Part model, mm, in its own coordinate system. Face numbers are marked on the shaded views. A direction names the side the tool comes from. Round coordinates to 2 decimals unless told otherwise and drop trailing zeros. Write each loop counter-clockwise with the first axis right and the second up, starting at its lowest first coordinate (ties: lowest second). Pieces come first, ordered by that corner, then holes. Notation, with made-up numbers: (-2, -37.75) -> (24, -37.75) arc R7 cw to (24, -25.75) -> close; hole circle Ø5 at (60.5, 13). An arc over 180 degrees is marked (long way). Use CSV: the item, a comma, the result in double quotes. Start each with the question number.
Autodesk Inventor part; units mm, degrees
ref_plane "YZ Plane" through (0, 0, 0) normal (1, 0, 0) x (0, 1, 0)
ref_plane "XZ Plane" through (0, 0, 0) normal (0, 1, 0) x (-1, 0, 0)
ref_plane "XY Plane" through (0, 0, 0) normal (0, 0, 1) x (1, 0, 0)
sketch "Skizze1" plane through (0, 0, 0) normal (0, 0, 1) x (1, 0, 0)
  arc A0 (-8.1406, -4.7) -> (-8.6412, -3.7) centre (0, 0) ccw
  line L0 (-18.5, -6.7) -> (-8.3427, -6.7)
  line L1 (-18.5, -6.7) -> (-18.5, -4.7)
  line L2 (-18.5, -4.7) -> (-8.1406, -4.7)
  line L3 (-18.5, -1.7) -> (-18.5, -3.7)
  line L4 (-18.5, -3.7) -> (-8.6412, -3.7)
  line L5 (-18.5, -1.7) -> (-14.519, -1.7)
  arc A1 (-8.3427, -6.7) -> (-10.5682, 1.6741) centre (0, 0) ccw
  arc A2 (-14.519, -1.7) -> (-10.5682, 1.6741) centre (-14.519, 2.3) ccw
  point P0 (-10.5641, -1.7)
  dimension "d0" = 18.8
  dimension "d2" = 2
  dimension "d4" = 1
  dimension "d5" = 18.5
  dimension "d6" = 4
  dimension "d7" = 1.3
  dimension "d19" = 10.1573
  dimension "d26" = 4
extrude "Extrusion1" add sketch "Skizze1" along normal mid plane 14
sketch "Skizze2" plane through (-18.5, -1.7, 7) normal (0, 1, 0) x (1, 0, 0)
  circle A0 centre (3, 11) radius 1.65
  line L0 (0, 14) -> (3.981, 14)
  line L1 (0, 14) -> (0, 0)
  line L2 (0, 14) -> (0, 0) construction
  line L3 (0, 7) -> (7.2294, 7) construction
  circle A1 centre (3, 3) radius 1.65
  circle A2 centre (3, 11) radius 3
  circle A3 centre (3, 3) radius 3
  point P0 (18.5, 7)
  point P1 (9.0709, 16)
  point P2 (0, 3)
  point P3 (0, 0.6676)
  point P4 (0.6676, 16)
  point P5 (0, 11)
  point P6 (0, 10.6676)
  point P7 (3, 14)
  dimension "d10" = 3
  dimension "d11" = 3
  dimension "d12" = 3.3
  dimension "d20" = 6
extrude "Extrusion2" cut sketch "Skizze2" against normal through all both and the other way through all contours A0 | A1
fillet "Rundung2" radius 4 1 edges at (-8.3427, -6.7, 0)
fillet "Rundung3" radius 0.8 2 edges at (-8.6412, -3.7, 0) (-8.1406, -4.7, 0)
extrude "Extrusion4" cut sketch "Skizze2" along normal blind 10 contours A3 | A2
properties part number "Halterung_Akku_210403"
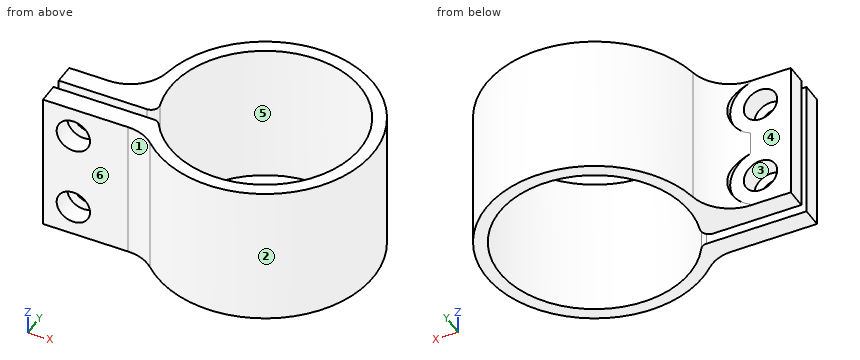
1. Band-saw the part on A-A (x = -15.5). List the corners of the cut face in (y, z).
2. Drill centre lines: line 1 along Z through (x, y) = (-15.5, -2.95); line 2 along X through (y, z) = (-3.1, -4); line 3 along X through (y, z) = (-5, 3). Where is each one in solid material? Low to high. Write a range as [from, to].
3. Band-saw the part on B-B (z = 4). List the corners of the cut face in (x, y), then the cut area to 3 significant figures.
4. Which spindle directions (+Z, -Z, +X, -X, +Y, -Y) get a long thin tool onto all of the face, cutting with end or side? Do the marked faces 4, 5 and 6. Say none if no direction does.
5. Pull direction X, two halves, no side cores. Call the marked faces 1, 2 and 3: released by +X, released by -X, zero draft, split by the parting line, or undercut.
6. Flat gauge pins, fed straight in: pin 1 (1.5 mm diameter, centred on y = 6.5, z = 5, fed in from -X); pin 2 (5 mm diameter, centred on x = 3, z = 4, fed in from +Y); pin 3 (5 mm diameter, centred on x = -5.5, z = -4.5, fed in from +Y). Where does each tip first touch, or does it go through?
7. Band-saw the part on D-D (x = -6.5). List the corners of the cut face in (y, z), then the cut area to 3 significant figures.
8. Band-saw the part on C-C (y = 2.25). List the corners of the cut face in (x, z), then the cut area to 3 significant figures.
Answers below:
1,outline,"(-6.7, -7) -> (-4.7, -7) -> (-4.7, -5.65) -> (-6.7, -5.65) -> close; (-6.7, -2.35) -> (-4.7, -2.35) -> (-4.7, 2.35) -> (-6.7, 2.35) -> close; (-6.7, 5.65) -> (-4.7, 5.65) -> (-4.7, 7) -> (-6.7, 7) -> close; (-3.7, -7) -> (-1.7, -7) -> (-1.7, -5.65) -> (-3.7, -5.65) -> close; (-3.7, -2.35) -> (-1.7, -2.35) -> (-1.7, 2.35) -> (-3.7, 2.35) -> close; (-3.7, 5.65) -> (-1.7, 5.65) -> (-1.7, 7) -> (-3.7, 7) -> close"
2,line 1,"z = [-7, -5.65], [-2.35, 2.35], [5.65, 7]"
2,line 2,"x = [-18.5, -17.15], [-13.85, -9], [8.87, 10.24]"
2,line 3,"x = [-18.5, -16.81], [-14.19, -7.97], [7.96, 9.46]"
3,outline,"(-18.5, -6.7) -> (-17.15, -6.7) -> (-17.15, -4.7) -> (-18.5, -4.7) -> close; (-18.5, -3.7) -> (-17.15, -3.7) -> (-17.15, -1.7) -> (-18.5, -1.7) -> close; (-13.85, -6.7) -> (-10.08, -6.7) arc R4 cw to (-7.34, -7.79) arc R10.7 ccw (long way) to (-10.57, 1.67) arc R4 cw to (-12.5, -1.15) -> (-12.5, -1.7) -> (-13.85, -1.7) -> (-13.85, -3.7) -> (-9.78, -3.7) arc R0.8 ccw to (-9.01, -2.67) arc R9.4 cw (long way) to (-7.92, -5.07) arc R0.8 ccw to (-8.59, -4.7) -> (-13.85, -4.7) -> close"
3,area,"105 mm^2"
4,face 4,"-X, +Y"
4,face 5,"+Z, -Z"
4,face 6,"+Z, -Z, -X, -Y"
5,face 1,"released by -X"
5,face 2,"split by the parting line"
5,face 3,"undercut"
6,pin 1,"stops at x = -9.02"
6,pin 2,"stops at y = 10.69"
6,pin 3,"stops at y = 10.27"
7,outline,"(-8.5, -7) -> (-6.79, -7) -> (-6.79, 7) -> (-8.5, 7) -> close; (6.79, -7) -> (8.5, -7) -> (8.5, 7) -> (6.79, 7) -> close"
7,area,"47.8 mm^2"
8,outline,"(-10.46, -7) -> (-9.13, -7) -> (-9.13, 7) -> (-10.46, 7) -> close; (9.13, -7) -> (10.46, -7) -> (10.46, 7) -> (9.13, 7) -> close"
8,area,"37.4 mm^2"
